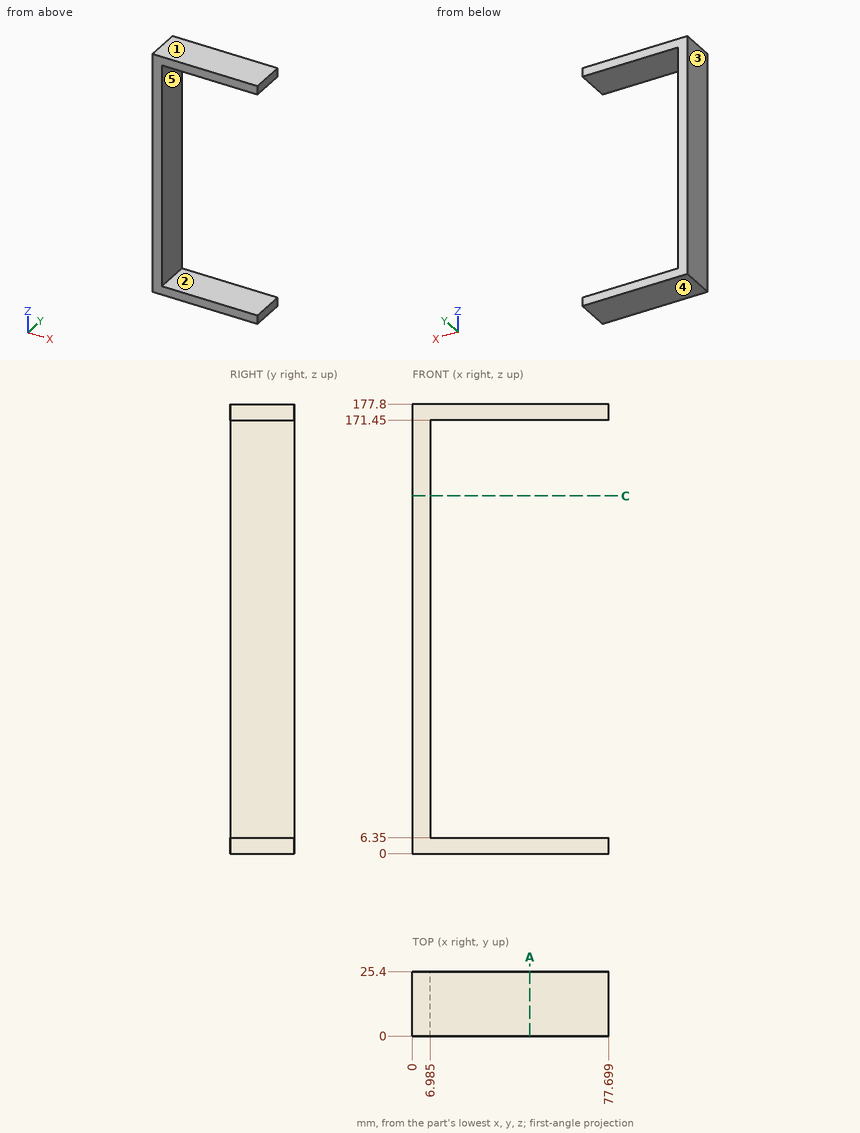
Answer from the drawing. Dimensions are ordinates in mm from the lowest x, y and z of the part. A direction names the side the tool comes from. Round coordinates to 2 decimals unless told otherwise and drop trailing zeros. Loops run counter-clockwise (first coordinate to the right, second up) from the corner with the lowest first, then second, coordinate; pieces in that order, holes last.
1) A cutting plane is placed at A-A on x = 46.5. Determine the outline of the cut face in (y, z).
Outcome:
outline: (0, 0) - (25.4, 0) - (25.4, 6.35) - (0, 6.35) - close; (0, 171.45) - (25.4, 171.45) - (25.4, 177.8) - (0, 177.8) - close
2) For a pull along Z with two mould halves and no side action, classify the marked faces 1, 2 and 3 as released by +Z, released by -Z, zero draft, split by the parting line, or undercut.
Outcome:
face 1: released by +Z
face 2: undercut
face 3: zero draft
3) A cutting plane is placed at C-C on z = 141.5. Determine the outline of the cut face in (x, y) (1 decimal), plus the area to 3 significant figures.
Outcome:
outline: (0, 0) - (7, 0) - (7, 25.4) - (0, 25.4) - close
area: 177 mm2
4) Consider line 1 (Z direction, x = 37, y = 22.5); line 2 (X direction, y = 8.5, z = 86.5) (1 decimal). Determine where each line is inside the solid, lowest interval first.
Outcome:
line 1: z = 0 to 6.35, 171.45 to 177.8
line 2: x = 0 to 7
5) Given P1, Ø3, axis at y = 10.5, z = 18, coming from the +X side (3 decimals), flat-ended and moving along its own axis, determine where the tip first touches the part or whether it passes through.
Outcome:
P1: stops at x = 6.985
6) For the marked faces 4 and 5, determine the directions among +Z, -Z, +X, -X, +Y, -Y from which every point of the face is accessible in a straight line to the end or side of a thin tool.
Outcome:
face 4: -Z, +X, -X, +Y, -Y
face 5: +X, +Y, -Y
